Could you check a few things on this drawing? It's one solid part, dimensions in mm from its lowest x, y, z. Give positions to 0.01 mm unless a question says otherwise; leave off trailing zeros. Order: outer loops, then holes, each group sorted by start corner. A loop starts at its lowest first (then second) coordinate and runs counter-clockwise, first axis right, second up. Notation, with made-up numbers: (28, 59) -> (74, 59) arc R4 cw to (74, 66) -> close; hole circle Ø11 at (51.5, -6.75). An arc over 180 degrees is marked (long way). Write each question's results on one line, items separated by ' | '. Start each with the question number.
Q1. Imagine slicing it at A-A, the plane y = 37. Please give me the cut outline in (x, z).
Q2. I need wall thicknesses on line 1 along Z through (x, y) = (29.5, 27); line 2 along Z through (x, y) = (38, 69); line 3 along Y through (x, z) = (10, 370.5). Which ranges of each line are inside material? Lowest first, please. Write a range as [from, to].
Q3. Imagine slicing it at D-D, the plane x = 11.5. Please give me the cut outline in (y, z).
Q4. Imagine slicing it at C-C, the plane z = 69.5. Please give me the cut outline in (x, y), then the cut area to 3 significant figures.
Q5. Imagine slicing it at B-B, the plane x = 45.5. Please give me the cut outline in (y, z), then the cut area to 3 significant figures.
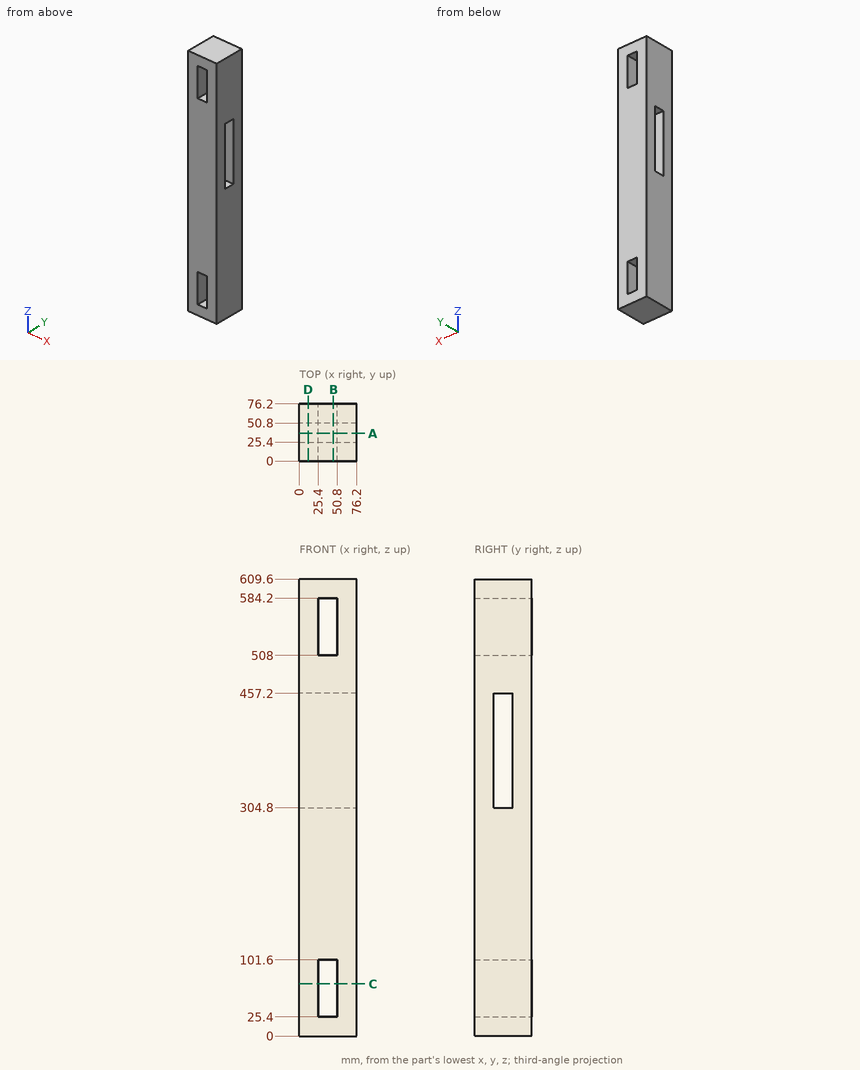
Geometry check:
1) outline: (0, 0) -> (76.2, 0) -> (76.2, 304.8) -> (0, 304.8) -> close; (0, 457.2) -> (76.2, 457.2) -> (76.2, 609.6) -> (0, 609.6) -> close; hole (25.4, 25.4) -> (50.8, 25.4) -> (50.8, 101.6) -> (25.4, 101.6) -> close; hole (25.4, 508) -> (50.8, 508) -> (50.8, 584.2) -> (25.4, 584.2) -> close
2) line 1: [0, 25.4], [101.6, 304.8], [457.2, 508], [584.2, 609.6] | line 2: [0, 25.4], [101.6, 508], [584.2, 609.6] | line 3: [0, 25.4], [50.8, 76.2]
3) outline: (0, 0) -> (76.2, 0) -> (76.2, 609.6) -> (0, 609.6) -> close; hole (25.4, 304.8) -> (50.8, 304.8) -> (50.8, 457.2) -> (25.4, 457.2) -> close
4) outline: (0, 0) -> (25.4, 0) -> (25.4, 76.2) -> (0, 76.2) -> close; (50.8, 0) -> (76.2, 0) -> (76.2, 76.2) -> (50.8, 76.2) -> close | area: 3,870 mm²
5) outline: (0, 0) -> (76.2, 0) -> (76.2, 25.4) -> (0, 25.4) -> close; (0, 101.6) -> (76.2, 101.6) -> (76.2, 508) -> (0, 508) -> close; (0, 584.2) -> (76.2, 584.2) -> (76.2, 609.6) -> (0, 609.6) -> close; hole (25.4, 304.8) -> (50.8, 304.8) -> (50.8, 457.2) -> (25.4, 457.2) -> close | area: 31,000 mm²
